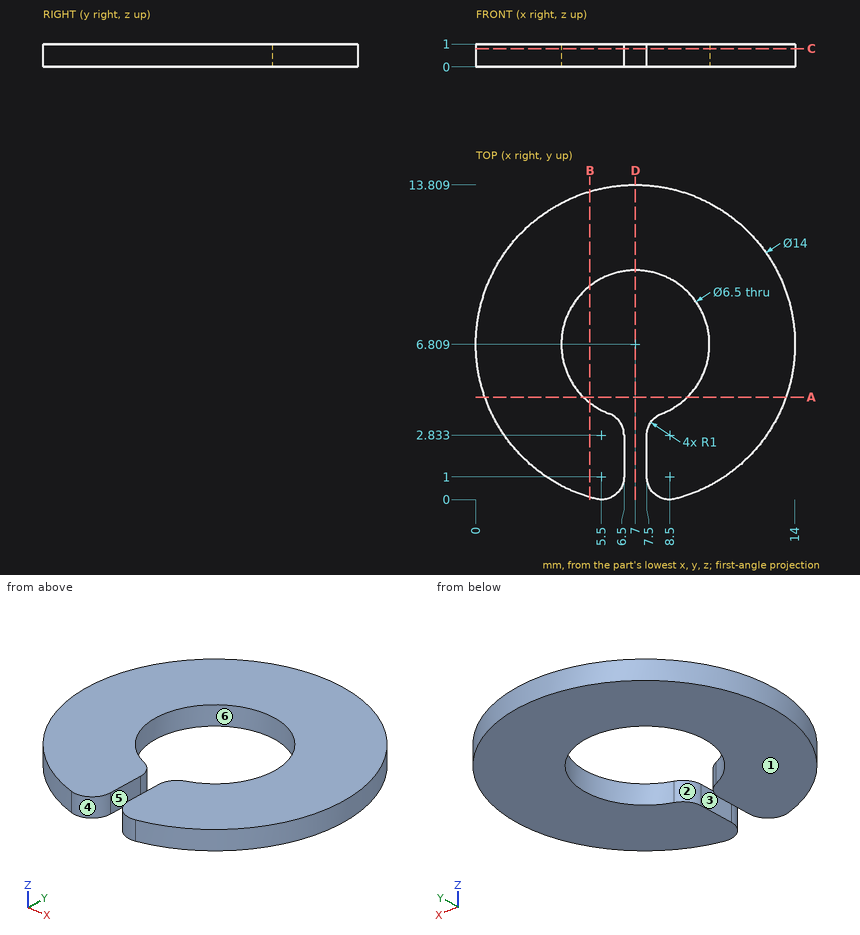
Job drawing, mm, ordinate dimensions from the low corner. One solid piece. A direction names the side the tool comes from. Coordinates: 2 decimals unless noted, no trailing zeros. Write each loop counter-clockwise with the first axis right and the second up, starting at its lowest first coordinate (ties: lowest second). Pieces come first, ordered by that corner, then holes. Notation, with made-up numbers: M -11.5,-27 L 42.5,-27 A33 ccw 42.5,12 Z; hole C -27.5,16 d10. An arc over 180 degrees is marked long. Answer as a JSON object with one key per item and string values. Group by question number.
1) Saw through at C-C (z = 0.8). Write the cut outline in (x, y), plus the area to 3 significant figures.
2) Saw through at D-D (x = 7). Write the cut outline in (y, z).
3) Wall check: line 1 (X direction, y = 3, z = 0.2) (1 decimal); line 2 (X direction, y = 6, z = 0.95); line 3 (Y direction, x = 5.5, z = 0.85) (1 decimal). Give the ranges that are in metal, low to high. Write a range as from..to.
4) Tool access for the marked faces 1, 2 and 3: list every direction of +Z, -Z, +X, -X, +Y, -Y with a clear straight run to the whole face (end or side of a thin tool).
5) Pin check, flat tip, straight feed: pin 1 Ø0.5 at (y, z) = (2, 0.5) entering from -X. Stop position of the tip, or through.
6) Saw through at B-B (x = 5). Write the cut outline in (y, z).
7) Mould opens along Y. For the marked faces 4, 5 and 6 say: +Y half, -Y half, draft (parallel to the pull), parting line (faces both ways), or undercut.
8) Saw through at A-A (y = 4.5). Write the cut outline in (x, z).
Values follow:
{
 "1": {"outline": "M 5.25,0.03 A1 ccw 6.5,1 L 6.5,2.83 A1 ccw 5.85,3.77 A3.25 cw long 8.15,3.77 A1 ccw 7.5,2.83 L 7.5,1 A1 ccw 8.75,0.03 A7 ccw long Z", "area": "116 mm2"},
 "2": {"outline": "M 10.06,0 L 13.81,0 L 13.81,1 L 10.06,1 Z"},
 "3": {"line 1": "x = 1.1..6.5, 7.5..12.9", "line 2": "x = 0.05..3.85, 10.15..13.95", "line 3": "y = 0..3.9, 9.7..13.6"},
 "4": {"face 1": "-Z, +X, -X, +Y, -Y", "face 2": "+Z, -Z", "face 3": "+Z, -Z, -Y"},
 "5": {"pin 1": "stops at x = 1.69"},
 "6": {"outline": "M 0.1,0 L 4.25,0 L 4.25,1 L 0.1,1 Z; M 9.37,0 L 13.52,0 L 13.52,1 L 9.37,1 Z"},
 "7": {"face 4": "-Y half", "face 5": "draft", "face 6": "undercut"},
 "8": {"outline": "M 0.39,0 L 4.71,0 L 4.71,1 L 0.39,1 Z; M 9.29,0 L 13.61,0 L 13.61,1 L 9.29,1 Z"}
}
